Source: three-view drawing plus pictorial views. Frame: mm from the lowest corner of the part. Round coordinates to 2 decimals unless told otherwise and drop trailing zeros. Write each loop counter-clockwise with the first axis right and the second up, starting at its lowest first coordinate (ties: lowest second). Pieces come first, ordered by that corner, then holes. Notation, with made-up numbers: M -21,89.5 L 17,89.5 A23 cw 17,113.5 Z; hole C 64.5,79 d1. An arc over 180 degrees is marked long. Answer as CSV lines item,"result". Start each with the question number.
Q1. Section query D-D on x = 7.5. Output: boundary loops of the cut face in (y, z), and give its area (3 significant figures).
Q2. Ray query, probe 1 along Y at (x, z) = (40, 3.05); probe 2 along Y at (x, z) = (41.5, 0.45); probe 3 along X at (y, z) = (14, 2.1) (1 decimal). Return the intervals inside material, ascending.
Q3. Section query C-C on z = 0.95. Output: boundary loops of the cut face in (x, y) (1 decimal), and give its area (3 significant figures).
Q4. Section query A-A on x = 40. Output: boundary loops of the cut face in (y, z).
Q5. First-contact query: pin 1 (1 mm diameter, centred on y = 34, z = 2.5, fed in from +X); pin 2 (1 mm diameter, centred on x = 68.5, z = 2.5, fed in from +Y) (1 decimal); pin 3 (3 mm diameter, centred on y = 62.5, z = 4, fed in from +X) (1 decimal). Flat tips, straight axial feed; report the tip coordinate or a pass-through.
Q6. Mould query, pull axis X, two halves, no side actions, for the marked faces 1, 2 and 3. Classes: pulls with the +X half, pulls with the -X half, needs draft (parallel to the pull), parting line crosses it, or undercut.
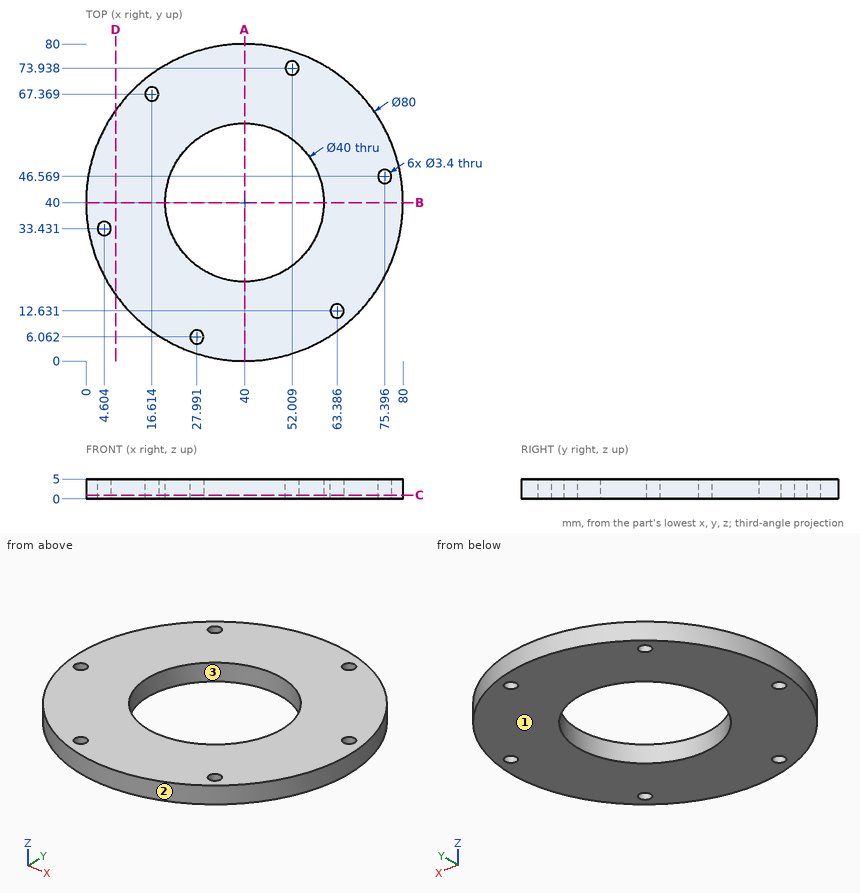
Entries:
1,outline,"M 16.68,0 L 63.32,0 L 63.32,5 L 16.68,5 Z"
1,area,"233 mm^2"
2,probe 1,"y = 0 to 20, 60 to 80"
2,probe 2,"y = 0.03 to 20.06, 59.94 to 79.97"
2,probe 3,"x = 9.6 to 62.4, 64.4 to 70.4"
3,outline,"C 40,40 d80; hole C 4.6,33.4 d3.4; hole C 16.6,67.4 d3.4; hole C 40,40 d40; hole C 28,6.1 d3.4; hole C 52,73.9 d3.4; hole C 63.4,12.6 d3.4; hole C 75.4,46.6 d3.4"
3,area,"3,720 mm^2"
4,outline,"M 0,0 L 20,0 L 20,5 L 0,5 Z; M 60,0 L 80,0 L 80,5 L 60,5 Z"
5,pin 1,"stops at x = 79.62"
5,pin 2,"stops at y = 68.6"
5,pin 3,"stops at x = 74"
6,face 1,"needs draft"
6,face 2,"parting line crosses it"
6,face 3,"undercut"
